The listing builds one solid part. Answer for the finished solid, in the listing's coordinates (mm). Give positions to 0.01 mm unless a question says otherwise; leave off trailing zeros. Loops run counter-clockwise (first coordinate to the right, second up) from the corner with the lowest first, then second, coordinate; pieces in that order, holes last. Notation, with made-up numbers: M 9.5,-38 L 18.5,-38 A15 ccw 18.5,-11 Z; hole C -32.75,-29 d5. An arc over 180 degrees is marked long. One line per item, written item: value. Start each with the question number.
Q1. A cutting plane is placed at B-B, the plane x = 36. Determine the outline of the cut face in (y, z).
Q2. A cutting plane is placed at A-A, the plane z = 42.5. Determine the outline of the cut face in (x, y).
Q3. Consider L1, parallel to X at y = 2.6, z = 35; L2, parallel to X at y = 3.45, z = 38; L3, parallel to Z at x = 60, y = 3.2. Determine where each line is inside the solid, lowest interval first.
Q4. Flat-ended cylindrical pins translate along their axes: pin 1 (3 mm diameter, centred on x = 55, y = 4, fed in from -Z); pin 2 (1.5 mm diameter, centred on y = 0.5, z = 25, fed in from +X); pin 3 (1 mm diameter, centred on y = 4, z = 39, fed in from +X). Find the tip coordinate at first contact, or state that the pin passes through.
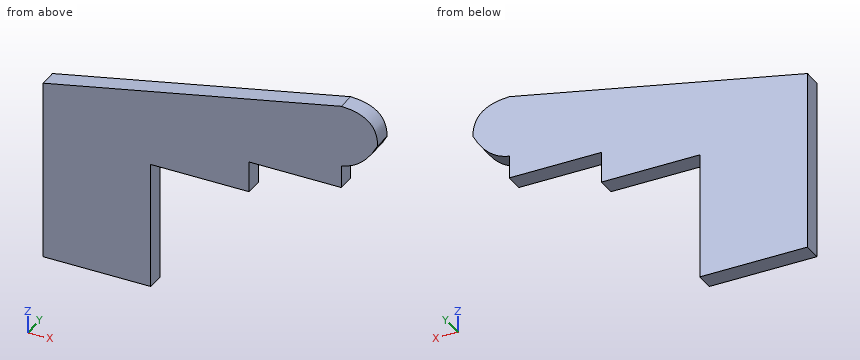
from build123d import *

# Parameters (mm, degrees)
BOSS_EXTRUDE2_DEPTH = 5.08


with BuildPart() as part:
    # Sketch2 → Boss-Extrude2 (new body)
    with BuildSketch(Plane(origin=(0, 0, 0), x_dir=(1, 0, 0), z_dir=(0, 1, 0))):
        with BuildLine():
            Line((0, 0), (30.130673801, 0))
            Line((30.130673801, 0), (30.130673801, -29.621601631))
            Line((30.130673801, -29.621601631), (30.130673801, -35.708970709))
            Line((30.130673801, -35.708970709), (57.668772007, -35.708970709))
            Line((57.668772007, -35.708970709), (57.668772007, -44.405212247))
            Line((57.668772007, -44.405212247), (83.467621906, -44.405212247))
            Line((83.467621906, -44.405212247), (83.467621906, -50.782456043))
            add(Edge.make_bspline(
                [(93.613237035, -59.478697582), (89.75401012, -51.849955928), (83.467621906, -50.782456043)],
                knots=[0, 0, 0, 0.754491666, 0.754491666, 0.754491666], degree=2))
            add(Edge.make_bspline(
                [(83.467621906, -68.17493912), (93.746562006, -67.908588045), (93.613237035, -59.478697582)],
                knots=[0, 0, 0, 1, 1, 1], degree=2))
            Line((83.467621906, -68.17493912), (0, -50.782456043))
            Line((0, -50.782456043), (0, 0))
        make_face()
    extrude(amount=BOSS_EXTRUDE2_DEPTH)


solid = part.part
Answer block:
1. outline: M 0,35.71 L 5.08,35.71 L 5.08,58.28 L 0,58.28 Z
2. outline: M 0,0 L 57.67,0 L 57.67,5.08 L 0,5.08 Z
3. L1: 0 to 30.13
3. L2: 0 to 57.67
3. L3: 44.41 to 63.28
4. pin 1: z = 35.71
4. pin 2: x = 30.13
4. pin 3: x = 57.67
